For this review, take the finished solid that the model builds, in its own axes (mm). Face numbers are marked on the shaded views. A direction names the side the tool comes from. Coordinates: 2 decimals unless noted, no trailing zeros. Write each loop counter-clockwise with the first axis right and the second up, starting at its lowest first coordinate (ties: lowest second). Pieces come first, ordered by that corner, then holes. Notation, with made-up numbers: M -4,-32.75 L 37,-32.75 A33 ccw 37,6.25 Z; hole C 30,-20.5 d5. An arc over 180 degrees is marked long. One line per question, with ' | ' between items.
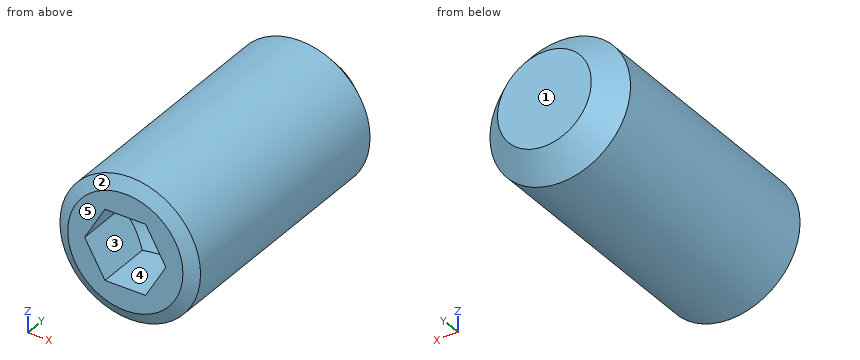
Solid Edge part; units mm, degrees
sketch "Sketch1" plane through (0, 0, 0) normal (0, 0, 1) x (1, 0, 0)
  line L0 (3, 10.6874) -> (3, 0)
  line L1 (2.4585, -0.3126) -> (3, 0)
  line L2 (0, -0.3126) -> (2.4585, -0.3126)
  line L3 (0, 0) -> (0, -0.3126)
  line L4 (0, 0) -> (0, 11.6874)
  line L5 (0, 11.6874) -> (2, 11.6874)
  line L6 (2, 11.6874) -> (3, 10.6874)
revolve "RevolvedProtrusion1" add sketch "Sketch1" angle 360 about axis through (0, 0, 0) along (0, 1, 0)
sketch "Sketch2" plane through (0, 0, 0) normal (0, 0, 1) x (1, 0, 0)
  line L0 (0, -0.3126) -> (0, 3.0392)
  line L1 (-2.3414, 1.6874) -> (0, 3.0392)
  line L2 (-2.3414, -0.3126) -> (-2.3414, 1.6874)
  line L3 (0, -0.3126) -> (-2.3414, -0.3126)
revolve "RevolvedCutout1" cut sketch "Sketch2" angle 360 about axis through (0, -0.1937, 0) along (0, 1, 0)
sketch "Sketch3" plane through (0, -0.3126, 0) normal (0, -1, 0) x (0, 0, -1)
  line L0 (-1.5, -0.866) -> (0, -1.7321)
  line L1 (0, -1.7321) -> (1.5, -0.866)
  line L2 (1.5, -0.866) -> (1.5, 0.866)
  line L3 (1.5, 0.866) -> (0, 1.7321)
  line L4 (0, 1.7321) -> (-1.5, 0.866)
  line L5 (-1.5, 0.866) -> (-1.5, -0.866)
  circle A0 centre (0, 0) radius 2.3414
extrude "Protrusion1" add sketch "Sketch3" against normal up to next
cosmetic_thread "Thread1"
1) The part is to be moulded in two halves that separate along X. For the marked faces 1, 2 and 3, say which applies: +X half, -X half, draft (parallel to the pull), parting line (faces both ways), or undercut.
Responses:
face 1: draft | face 2: parting line | face 3: undercut
2) Machinability: for the marked faces 4 and 5, which of the approach directions +Z, -Z, +X, -X, +Y, -Y give a long, thin tool a straight path to every point of the face, cutting with its end or side? Answer none if there is none.
Responses:
face 4: -Y | face 5: +Z, -Z, +X, -X, -Y
3) To check wall thickness, follow line 1 along Z through (x, y) = (0.6, 2.5); line 2 along X through (y, z) = (1.25, 0.5); line 3 along Z through (x, y) = (-1, 0.75). State the ranges of each line that lie inside material, in increasing order. Write a range as [from, to].
Responses:
line 1: [-2.94, -0.72], [0.72, 2.94] | line 2: [-2.96, -1.44], [1.44, 2.96] | line 3: [-2.83, -1.27], [1.27, 2.83]
4) Insertion check: pin 1 Ø3 at (y, z) = (4, -2) entering from +X; pin 2 Ø2 at (x, y) = (1.5, 3) entering from +Z. Each pin has a flat end and moves straight along its axis. Give the tip position at first contact, or say it passes through.
Responses:
pin 1: x = 2.96 | pin 2: z = 2.96
5) We need section A-A on y = 7.75. State the section outline as (x, z) points.
Responses:
outline: C 0,0 d6
